Geometry check sheet. Reference: the model listing, model coordinates, mm. A direction names the side the tool comes from. Give positions to 0.01 mm unless a question says otherwise; leave off trailing zeros. Loops run counter-clockwise (first coordinate to the right, second up) from the corner with the lowest first, then second, coordinate; pieces in that order, holes last. Notation, with made-up numbers: (27, 28.5) -> (40, 28.5) arc R11 cw to (40, 33.5) -> close; hole circle Ø5 at (42, -13.5). An arc over 180 degrees is marked (long way). One line per item, written item: value. Start each with the question number.
(1) Sectioned sample at B-B, the plane x = 18. Record the cut outline in (y, z).
(2) Gauge pin test, flat ends, axial feed: pin 1 Ø2.5 at (x, y) = (19.39, 5) entering from +Z; pin 2 Ø5 at (x, y) = (-13, 4) entering from +Z; pin 3 Ø4 at (y, z) = (3, 36) entering from -X; pin 4 Ø3 at (y, z) = (3, 26) entering from +X. Record the tip position at first contact, or that the pin passes through.
(3) Sectioned sample at A-A, the plane z = 28.5. Record the cut outline in (x, y).
(4) Scan lines: line 1 along X through (y, z) = (6.75, -9.5); line 2 along Z through (x, y) = (-15, 3.5); line 3 along Z through (x, y) = (3.5, 3.75). Record each from-to range of solid material in increasing order. Write a range as from..to.
(5) Sectioned sample at D-D, the plane x = 6. Record the cut outline in (y, z), then the cut area to 3 significant figures.
(6) Draft check along Z on faces 5 (the face through (-14.3, 2.7, -11.278)), 6 (the face through (-10, 5, -14.278)), 7 (the face through (12.91, 4.64, 19.72)), 8 (the face through (-6.59, 4.64, 19.72)). Enter one of: pulls with the +Z half, pulls with the -Z half, needs draft (parallel to the pull), parting line crosses it, or undercut.
(7) Tool access check on faces 1 (the face through (11.389, 7, 18)), 2 (the face through (24.389, 5, -13)), 3 (the face through (22, 5, -11.278)), 4 (the face through (-8.111, 5, 22)). Record the directions out of +Z, -Z, +X, -X, +Y, -Y that give a thin tool (end or side, any length) a straight path to the whole face; none if there is none.
(8) Sectioned sample at C-C, the plane y = 8. Record the cut outline in (x, z), then the cut area to 4 significant figures.
Autodesk Inventor part; units mm, degrees
ref_plane "YZ Plane" through (0, 0, 0) normal (1, 0, 0) x (0, 1, 0)
ref_plane "XZ Plane" through (0, 0, 0) normal (0, 1, 0) x (-1, 0, 0)
ref_plane "XY Plane" through (0, 0, 0) normal (0, 0, 1) x (1, 0, 0)
sketch "Sketch1" plane through (0, 0, 0) normal (0, 1, 0) x (-1, 0, 0)
  line L0 (-14.3889, -14.2778) -> (-11.3889, -14.2778)
  line L1 (-11.3889, -14.2778) -> (-11.3889, 54.2222)
  line L2 (-11.3889, 54.2222) -> (-14.3889, 54.2222)
  line L3 (-14.3889, 54.2222) -> (-14.3889, -14.2778)
  line L4 (-11.3889, 54.2222) -> (5.1111, 54.2222)
  line L5 (5.1111, 54.2222) -> (5.1111, 51.2222)
  line L6 (5.1111, 51.2222) -> (-11.3889, 51.2222)
  line L7 (-11.3889, 51.2222) -> (-11.3889, 54.2222)
  line L8 (5.1111, 54.2222) -> (8.1111, 54.2222)
  line L9 (8.1111, 54.2222) -> (8.1111, -14.2778)
  line L10 (8.1111, -14.2778) -> (5.1111, -14.2778)
  line L11 (5.1111, -14.2778) -> (5.1111, 54.2222)
  line L12 (8.1111, -14.2778) -> (18.1111, -14.2778)
  line L13 (18.1111, -14.2778) -> (18.1111, -11.2778)
  line L14 (18.1111, -11.2778) -> (8.1111, -11.2778)
  line L15 (8.1111, -11.2778) -> (8.1111, -14.2778)
  line L16 (-14.3889, -14.2778) -> (-24.3889, -14.2778)
  line L17 (-24.3889, -14.2778) -> (-24.3889, -11.2778)
  line L18 (-24.3889, -11.2778) -> (-14.3889, -11.2778)
  line L19 (-14.3889, -11.2778) -> (-14.3889, -14.2778)
  point P0 (0, 0)
  dimension "d0" = 10
  dimension "d1" = 10
  dimension "d2" = 3
  dimension "d3" = 3
  dimension "d4" = 3
  dimension "d5" = 3
  dimension "d6" = 3
  dimension "d7" = 68.5
  dimension "d8" = 16.5
extrude "Extrusion1" add sketch "Sketch1" along normal blind 10
sketch "Sketch2" plane through (14.3889, 0, 54.2222) normal (1, 0, 0) x (0, 0, -1)
  line L0 (0, 10) -> (65.5, 10)
  line L1 (0, 0) -> (65.5, 0)
  line L2 (31.75, 14.4261) -> (31.75, -5.3494)
  line L3 (68.5, 0) -> (68.5, 10)
  circle A0 centre (36.75, 4.5383) radius 2.25
  line L4 (31.75, 4.5383) -> (48.4854, 4.5383)
  point P0 (54.2222, 0)
  dimension "d11" = 36.75
  dimension "d12" = 4.5
  dimension "d13" = 5
extrude "Extrusion2" cut sketch "Sketch2" against normal blind 40
sketch "Sketch3" plane through (14.3889, 0, -11.2778) normal (0, 0, 1) x (1, 0, 0)
  circle A0 centre (5, 5) radius 2.25
  point P0 (-14.3889, 0)
  dimension "d16" = 4.5
extrude "Extrusion3" cut sketch "Sketch3" against normal blind 3
sketch "Sketch4" plane through (-18.1111, 0, -11.2778) normal (0, 0, 1) x (1, 0, 0)
  circle A0 centre (5, 5) radius 2.25
  point P0 (18.1111, 0)
  dimension "d19" = 4.5
extrude "Extrusion4" cut sketch "Sketch4" against normal blind 3
properties part number "BarClip"
Calculated:
1. outline: (0, -14.28) -> (3.23, -14.28) -> (3.23, -11.28) -> (0, -11.28) -> close; (6.77, -14.28) -> (10, -14.28) -> (10, -11.28) -> (6.77, -11.28) -> close
2. pin 1: passes through
2. pin 2: stops at z = -11.28
2. pin 3: stops at x = -8.11
2. pin 4: stops at x = 14.39
3. outline: (-8.11, 0) -> (-5.11, 0) -> (-5.11, 10) -> (-8.11, 10) -> close; (11.39, 0) -> (14.39, 0) -> (14.39, 10) -> (11.39, 10) -> close
4. line 1: x = -8.11..-5.11, 11.39..14.39
4. line 2: z = -14.28..-11.28
4. line 3: z = 51.22..54.22
5. outline: (0, 51.22) -> (10, 51.22) -> (10, 54.22) -> (0, 54.22) -> close
5. area: 30.0 mm2
6. face 5: pulls with the +Z half
6. face 6: pulls with the -Z half
6. face 7: undercut
6. face 8: undercut
7. face 1: -Z, +Y, -Y
7. face 2: +Z, -Z, +X, +Y, -Y
7. face 3: +Z, +X, +Y, -Y
7. face 4: +Z, -X, +Y, -Y
8. outline: (-18.11, -14.28) -> (-5.11, -14.28) -> (-5.11, 51.22) -> (11.39, 51.22) -> (11.39, -14.28) -> (24.39, -14.28) -> (24.39, -11.28) -> (14.39, -11.28) -> (14.39, 54.22) -> (-8.11, 54.22) -> (-8.11, -11.28) -> (-18.11, -11.28) -> close
8. area: 520.5 mm2
